Print and shaded views of the part. All mm, measured from the part's lowest x, y and z. Give positions to 0.01 mm unless a question says otherwise; leave off trailing zeros. Loops run counter-clockwise (first coordinate to the right, second up) from the corner with the lowest first, then second, coordinate; pieces in that order, holes last.
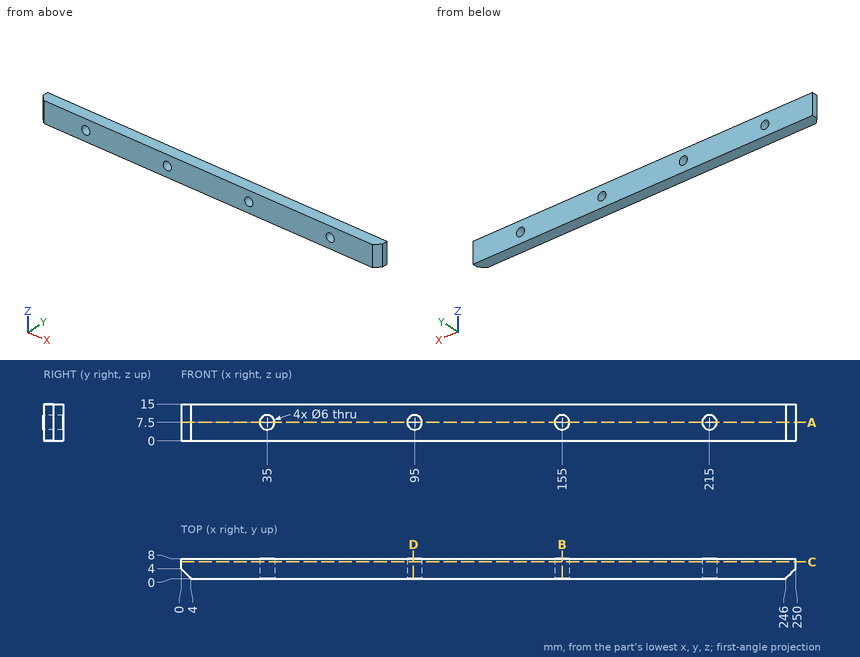
1. Drop flat-ended pins along their axis: pin 1 (3.5 mm diameter, centred on x = 95, z = 7.5, fed in from -Y) (3 decimals); pin 2 (1.5 mm diameter, centred on y = 1, z = 3.5, fed in from +X); pin 3 (1 mm diameter, centred on x = 137.5, z = 10, fed in from -Y). Give the stop position or say it passes through.
Responses:
pin 1: passes through
pin 2: stops at x = 247.75
pin 3: stops at y = 0
2. Saw through at A-A, the plane z = 7.5. List the corners of the cut face in (x, y).
Responses:
outline: (0, 4) - (4, 0) - (32, 0) - (32, 8) - (0, 8) - close; (38, 0) - (92, 0) - (92, 8) - (38, 8) - close; (98, 0) - (152, 0) - (152, 8) - (98, 8) - close; (158, 0) - (212, 0) - (212, 8) - (158, 8) - close; (218, 0) - (246, 0) - (250, 4) - (250, 8) - (218, 8) - close
3. Saw through at B-B, the plane x = 155. List the corners of the cut face in (y, z).
Responses:
outline: (0, 0) - (8, 0) - (8, 4.5) - (0, 4.5) - close; (0, 10.5) - (8, 10.5) - (8, 15) - (0, 15) - close
4. Probe line 1 along Z through (x, y) = (155, 2); line 2 along Z through (x, y) = (214, 5.25); line 3 along X through (y, z) = (5.75, 9.25). List the from-to ranges inside material, lowest first.
Responses:
line 1: z = 0 to 4.5, 10.5 to 15
line 2: z = 0 to 4.67, 10.33 to 15
line 3: x = 0 to 32.56, 37.44 to 92.56, 97.44 to 152.56, 157.44 to 212.56, 217.44 to 250
5. Saw through at C-C, the plane y = 6.75. List the corners of the cut face in (x, z).
Responses:
outline: (0, 0) - (250, 0) - (250, 15) - (0, 15) - close; hole circle Ø6 at (35, 7.5); hole circle Ø6 at (95, 7.5); hole circle Ø6 at (155, 7.5); hole circle Ø6 at (215, 7.5)
6. Saw through at D-D, the plane x = 94.5. List the corners of the cut face in (y, z).
Responses:
outline: (0, 0) - (8, 0) - (8, 4.54) - (0, 4.54) - close; (0, 10.46) - (8, 10.46) - (8, 15) - (0, 15) - close
